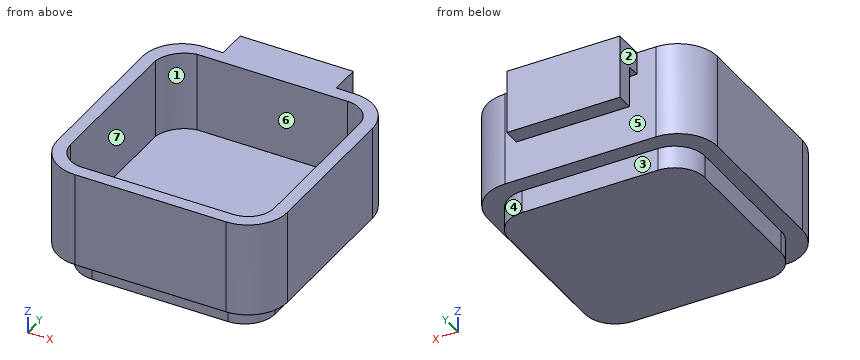
from build123d import *

# Parameters (mm, degrees)
F0_W     = 7
F0_H     = 40
F0_W_2   = 40
F0_H_2   = 7
F1_DEPTH = 4
F0_H_3   = 3.5
F0_W_3   = 3.5
F2_DEPTH = 25
F3_W     = 30
F3_H     = 17
F4_DEPTH = 8
F5_W     = 3.5
F5_H     = 11
F6_DEPTH = 33
F7_W     = 52
F7_H     = 52
F8_DEPTH = 6
F9_R     = 8


with BuildPart() as f1:
    # F0 (on Top) → F1 (new body)
    with BuildSketch(Plane.XY):
        with Locations((-23.5, 0)):
            Rectangle(F0_W, F0_H)
        with BuildLine():
            Line((-27, 20), (-20, 20))
            Line((-20, 20), (-20, 27))
            ThreePointArc((-20, 27), (-24.5803009352, 24.5803009352), (-27, 20))
        make_face()
        with Locations((0, 23.5)):
            Rectangle(F0_W_2, F0_H_2)
        Rectangle(F0_W_2, F0_H)
        with BuildLine():
            Line((20, 20), (27, 20))
            ThreePointArc((27, 20), (24.9497474683, 24.9497474683), (20, 27))
            Line((20, 27), (20, 20))
        make_face()
        with Locations((23.5, 0)):
            Rectangle(F0_W, F0_H)
        with Locations((0, -23.5)):
            Rectangle(F0_W_2, F0_H_2)
        with BuildLine():
            Line((20, -20), (20, -27))
            ThreePointArc((20, -27), (24.9497474683, -24.9497474683), (27, -20))
            Line((27, -20), (20, -20))
        make_face()
        with BuildLine():
            ThreePointArc((-27, -20), (-24.9497474683, -24.9497474683), (-20, -27))
            Line((-20, -27), (-20, -20))
            Line((-20, -20), (-27, -20))
        make_face()
    extrude(amount=F1_DEPTH)

    # F0 (on Top) → F2 (join)
    with BuildSketch(Plane.XY):
        with BuildLine():
            Line((20, -27), (20, -30.5))
            ThreePointArc((20, -30.5), (27.4246212025, -27.4246212025), (30.5, -20))
            Line((30.5, -20), (27, -20))
            Line((27, -20), (27, -27))
            Line((27, -27), (20, -27))
        make_face()
        with BuildLine():
            ThreePointArc((27, -20), (24.9497474683, -24.9497474683), (20, -27))
            Line((20, -27), (27, -27))
            Line((27, -27), (27, -20))
        make_face()
        with Locations((0, -28.75)):
            Rectangle(F0_W_2, F0_H_3)
        with BuildLine():
            ThreePointArc((-30.5, -20), (-27.4246212025, -27.4246212025), (-20, -30.5))
            Line((-20, -30.5), (-20, -27))
            Line((-20, -27), (-27, -27))
            Line((-27, -27), (-27, -20))
            Line((-27, -20), (-30.5, -20))
        make_face()
        with BuildLine():
            Line((-27, -27), (-20, -27))
            ThreePointArc((-20, -27), (-24.9497474683, -24.9497474683), (-27, -20))
            Line((-27, -20), (-27, -27))
        make_face()
        with Locations((-28.75, 0)):
            Rectangle(F0_W_3, F0_H)
        with BuildLine():
            ThreePointArc((-20, 30.5), (-27.4246212025, 27.4246212025), (-30.5, 20))
            Line((-30.5, 20), (-27, 20))
            Line((-27, 20), (-27, 27))
            Line((-27, 27), (-20, 27))
            Line((-20, 27), (-20, 30.5))
        make_face()
        with BuildLine():
            Line((-27, 27), (-27, 20))
            ThreePointArc((-27, 20), (-24.5803009352, 24.5803009352), (-20, 27))
            Line((-20, 27), (-27, 27))
        make_face()
        with Locations((0, 28.75)):
            Rectangle(F0_W_2, F0_H_3)
        with BuildLine():
            Line((27, 20), (30.5, 20))
            ThreePointArc((30.5, 20), (27.4246212025, 27.4246212025), (20, 30.5))
            Line((20, 30.5), (20, 27))
            Line((20, 27), (27, 27))
            Line((27, 27), (27, 20))
        make_face()
        with BuildLine():
            ThreePointArc((20, 27), (24.9497474683, 24.9497474683), (27, 20))
            Line((27, 20), (27, 27))
            Line((27, 27), (20, 27))
        make_face()
        with Locations((28.75, 0)):
            Rectangle(F0_W_3, F0_H)
    extrude(amount=F2_DEPTH)

    # F3 (on face) → F4 (join)
    with BuildSketch(Plane(origin=(0, 30.5, 0), x_dir=(-1, 0, 0), z_dir=(0, 1, 0))):
        with Locations((0, 16.5)):
            Rectangle(F3_W, F3_H)
    extrude(amount=F4_DEPTH)

    # F5 (on face) → F6 (cut)
    with BuildSketch(Plane(origin=(-15, 0, 0), x_dir=(0, -1, 0), z_dir=(-1, 0, 0))):
        with Locations((-32.25, 13.5)):
            Rectangle(F5_W, F5_H)
    extrude(amount=-F6_DEPTH, mode=Mode.SUBTRACT)

    # F7 (on face) → F8 (join)
    with BuildSketch(Plane(origin=(0, 0, 0), x_dir=(1, 0, 0), z_dir=(0, 0, -1))):
        Rectangle(F7_W, F7_H)
    extrude(amount=F8_DEPTH)

    # F9
    f9_edges = [f1.edges().sort_by_distance(p)[0] for p in [
        (-26, -26, -3),
        (26, -26, -3),
        (26, 26, -3),
        (-26, 26, -3),
    ]]
    fillet(f9_edges, radius=F9_R)


solid = f1.part
Geometry check sheet. Reference: the model listing, model coordinates, mm. Face numbers are marked on the shaded views. A direction names the side the tool comes from. Give positions to 0.01 mm unless a question says otherwise; leave off trailing zeros. Order: outer loops, then holes, each group sorted by start corner. A loop starts at its lowest first (then second) coordinate and runs counter-clockwise, first axis right, second up. Notation, with made-up numbers: M 48.25,74 L 62.25,74 A31 ccw 62.25,113 Z; hole C -37,-26 d4. An arc over 180 degrees is marked long. Use a Markdown table: item, result.
Item 1: Depth check by flat-ended pin: P1, Ø6.5, axis at y = 34.5, z = 20.5, coming from the -X side; P2, Ø3, axis at y = -6, z = -4.5, coming from the +X side; P3, Ø5, axis at x = 7.5, z = -3, coming from the +Y side. Enter the tip coordinate at first touch or a pass-through.
Answers follow:
| item | result |
|---|---|
| P1 | stops at x = -15 |
| P2 | stops at x = 26 |
| P3 | stops at y = 26 |
Item 2: Material ranges on line 1 along Y through (x, z) = (-1.5, 22); line 2 along X through (y, z) = (12, 20.5); line 3 along Y through (x, z) = (20.5, 4.5), recorded low to high.
Answers follow:
| item | result |
|---|---|
| line 1 | y = -30.5 to -27, 27 to 38.5 |
| line 2 | x = -30.5 to -27, 27 to 30.5 |
| line 3 | y = -30.49 to -26.98, 26.98 to 30.49 |
Item 3: Section check C-C (y = -1). Record the cut outline in (x, z).
Answers follow:
| item | result |
|---|---|
| outline | M -30.5,0 L -26,0 L -26,-6 L 26,-6 L 26,0 L 30.5,0 L 30.5,25 L 27,25 L 27,4 L -27,4 L -27,25 L -30.5,25 Z |
Item 4: Section check B-B (z = 6). Record the cut outline in (x, y).
Answers follow:
| item | result |
|---|---|
| outline | M -30.5,-20 A10.5 ccw -20,-30.5 L 20,-30.5 A10.5 ccw 30.5,-20 L 30.5,20 A10.5 ccw 20,30.5 L -20,30.5 A10.5 ccw -30.5,20 Z; hole M -27,-20 A7 ccw -20,-27 L 20,-27 A7 ccw 27,-20 L 27,20 A7 ccw 20,27 L -20,27 A8.78 ccw -27,20 Z |
Item 5: Section check A-A (z = 17.5). Record the cut outline in (x, y), and give its area (3 significant figures).
Answers follow:
| item | result |
|---|---|
| outline | M -30.5,-20 A10.5 ccw -20,-30.5 L 20,-30.5 A10.5 ccw 30.5,-20 L 30.5,20 A10.5 ccw 20,30.5 L -20,30.5 A10.5 ccw -30.5,20 Z; M -15,34 L 15,34 L 15,38.5 L -15,38.5 Z; hole M -27,-20 A7 ccw -20,-27 L 20,-27 A7 ccw 27,-20 L 27,20 A7 ccw 20,27 L -20,27 A8.78 ccw -27,20 Z |
| area | 891 mm2 |
Item 6: Tool access check on the marked faces 1, 2 and 3. Record the directions out of +Z, -Z, +X, -X, +Y, -Y that give a thin tool (end or side, any length) a straight path to the whole face; none if there is none.
Answers follow:
| item | result |
|---|---|
| face 1 | +Z |
| face 2 | +Z, -Z, -X, +Y |
| face 3 | -Z, +X, -X, +Y |
Item 7: Section check D-D (z = -1). Record the cut outline in (x, y), and give its area (3 significant figures).
Answers follow:
| item | result |
|---|---|
| outline | M -26,-18 A8 ccw -18,-26 L 18,-26 A8 ccw 26,-18 L 26,18 A8 ccw 18,26 L -18,26 A8 ccw -26,18 Z |
| area | 2,650 mm2 |
Item 8: Draft check along X on the marked faces 4, 5, 6 and 7. Enter one of: +X half, -X half, draft (parallel to the pull), parting line (faces both ways), or undercut.
Answers follow:
| item | result |
|---|---|
| face 4 | +X half |
| face 5 | draft |
| face 6 | undercut |
| face 7 | undercut |
